Check sheet for the drawn part. Datum: minimum x, y, z corner. Units: mm. A direction names the side the tool comes from. Coordinates: 2 decimals unless noted, no trailing zeros. Write each loop counter-clockwise with the first axis right and the second up, starting at its lowest first coordinate (ties: lowest second). Pieces come first, ordered by that corner, then holes. Notation, with made-up numbers: (-13.5, -14) - (0.5, -14) arc R20 ccw to (0.5, 0) - close; hole circle Ø1 at (-20.75, -9). An arc over 180 degrees is marked (long way). Use one line per item in the form item = value. Start each with the question number.
1. Scan lines: line 1 along X through (y, z) = (33, 3.5); line 2 along X through (y, z) = (71, 22); line 3 along Y through (x, z) = (51, 43). Record each from-to range of solid material in increasing order.
2. Cross-section at B-B on z = 8. Record the boundary of the cut face in (x, y), then the cut area to 3 significant figures.
3. Draft check along Y on the marked faces 4, 5, 6 and 7. Enter one of: +Y half, -Y half, draft (parallel to the pull), parting line (faces both ways), or undercut.
4. Cross-section at A-A on x = 60. Record the boundary of the cut face in (y, z).
5. Go/stop test with flat-tipped pins: pin 1 Ø1.5 at (y, z) = (29, 22) entering from -X; pin 2 Ø12 at (x, y) = (13.5, 56) entering from +Z; pin 3 Ø5 at (y, z) = (25.5, 20.5) entering from +X. Record where each tip stops, or that it passes through.
6. Tool access check on the marked faces 1, 2 and 3. Record the directions out of +Z, -Z, +X, -X, +Y, -Y that give a thin tool (end or side, any length) a straight path to the whole face; none if there is none.
7. Cross-section at D-D on y = 5.5. Record the boundary of the cut face in (x, z), then the cut area to 3 significant figures.
8. Cross-section at C-C on y = 53.5. Record the boundary of the cut face in (x, z).
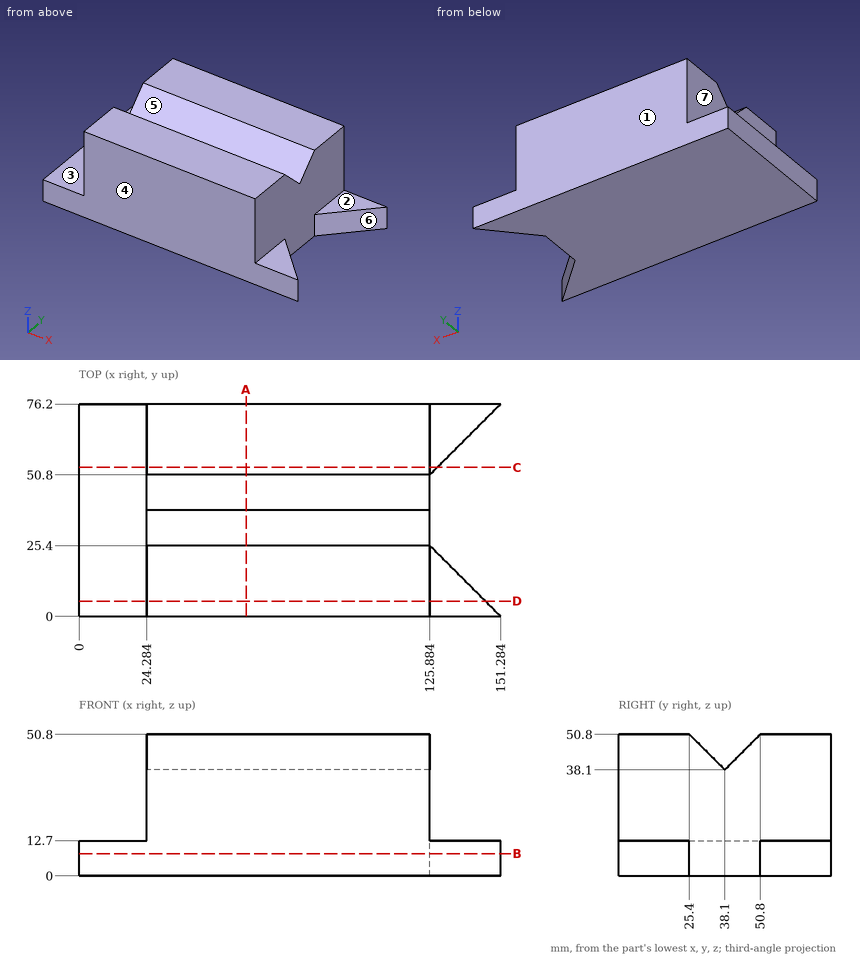
Final values:
q1.line_1 = 0 to 125.88
q1.line_2 = 24.28 to 125.88
q1.line_3 = 0 to 33.2, 43 to 76.2
q2.outline = (0, 0) - (151.28, 0) - (125.88, 25.4) - (125.88, 50.8) - (151.28, 76.2) - (0, 76.2) - close
q2.area = 10,200 mm²
q3.face_4 = -Y half
q3.face_5 = undercut
q3.face_6 = undercut
q3.face_7 = draft
q4.outline = (0, 0) - (76.2, 0) - (76.2, 50.8) - (50.8, 50.8) - (38.1, 38.1) - (25.4, 50.8) - (0, 50.8) - close
q5.pin_1 = 24.28
q5.pin_2 = 12.7
q5.pin_3 = 125.88
q6.face_1 = +Z, -Z, +X, -X, +Y
q6.face_2 = +Z, +X, +Y, -Y
q6.face_3 = +Z, -X, +Y, -Y
q7.outline = (0, 0) - (145.78, 0) - (145.78, 12.7) - (125.88, 12.7) - (125.88, 50.8) - (24.28, 50.8) - (24.28, 12.7) - (0, 12.7) - close
q7.area = 5,720 mm²
q8.outline = (0, 0) - (128.58, 0) - (128.58, 12.7) - (125.88, 12.7) - (125.88, 50.8) - (24.28, 50.8) - (24.28, 12.7) - (0, 12.7) - close
